from build123d import *

# Parameters (mm, degrees)
F1_W      = 200
F1_H      = 200
F1_W_2    = 191
F1_H_2    = 191
F2_DEPTH  = 94
F0_W      = 191
F0_H      = 191
F3_DEPTH  = 4
F6_W      = 20
F6_H      = 40
F9_DEPTH  = 35
F5_W      = 20
F5_H      = 40
F10_DEPTH = 35
F8_W      = 20
F8_H      = 40
F11_DEPTH = 35
F7_W      = 20
F7_H      = 40
F12_DEPTH = 35
F14_DEPTH = 25
F16_DEPTH = 25


with BuildPart() as f2:
    # F1 (on face) → F2 (new body)
    with BuildSketch(Plane.XY):
        Rectangle(F1_W, F1_H)
        Rectangle(F1_W_2, F1_H_2, mode=Mode.SUBTRACT)
    extrude(amount=F2_DEPTH)

    # F0 (on Top) → F3 (join)
    with BuildSketch(Plane.XY):
        Rectangle(F0_W, F0_H)
    extrude(amount=F3_DEPTH)

    # F6 (on offset) → F9 (join)
    with BuildSketch(Plane.XY.offset(39)):
        with Locations((-85.5, 75.5)):
            Rectangle(F6_W, F6_H)
    extrude(amount=-F9_DEPTH)

    # F5 (on offset) → F10 (join)
    with BuildSketch(Plane.XY.offset(39)):
        with Locations((-85.5, -75.5)):
            Rectangle(F5_W, F5_H)
    extrude(amount=-F10_DEPTH)

    # F8 (on offset) → F11 (join)
    with BuildSketch(Plane.XY.offset(39)):
        with Locations((85.5, -75.5)):
            Rectangle(F8_W, F8_H)
    extrude(amount=-F11_DEPTH)

    # F7 (on offset) → F12 (join)
    with BuildSketch(Plane.XY.offset(39)):
        with Locations((85.5, 75.5)):
            Rectangle(F7_W, F7_H)
    extrude(amount=-F12_DEPTH)

    # F13 (on face) → F14 (cut)
    with BuildSketch(Plane(origin=(-100, 0, 0), x_dir=(0, -1, 0), z_dir=(-1, 0, 0))):
        with BuildLine():
            Line((-67, 72), (-73, 72))
            ThreePointArc((-73, 72), (-77.949747, 69.949747), (-80, 65))
            Line((-80, 65), (-80, 52))
            Line((-80, 52), (-60, 52))
            Line((-60, 52), (-60, 65))
            ThreePointArc((-60, 65), (-62.050253, 69.949747), (-67, 72))
        make_face()
    extrude(amount=-F14_DEPTH, mode=Mode.SUBTRACT)

    # F15 (on face) → F16 (cut)
    with BuildSketch(Plane.YZ.offset(100)):
        with BuildLine():
            Line((-14, 62), (-16, 62))
            ThreePointArc((-16, 62), (-18.828427, 60.828427), (-20, 58))
            Line((-20, 58), (-20, 52))
            Line((-20, 52), (-10, 52))
            Line((-10, 52), (-10, 58))
            ThreePointArc((-10, 58), (-11.171573, 60.828427), (-14, 62))
        make_face()
    extrude(amount=-F16_DEPTH, mode=Mode.SUBTRACT)


solid = f2.part
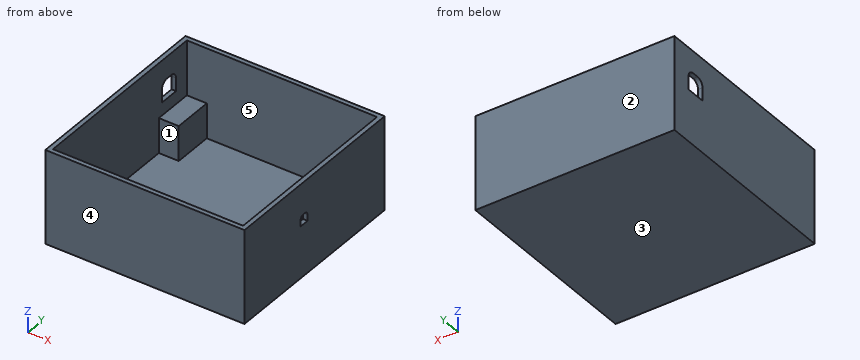
Input: part model. Units: mm. Frame: model coordinates. Face numbers are marked on the shaded views. A direction names the side the tool comes from. Give positions to 0.01 mm unless a question says otherwise; leave off trailing zeros. Write each loop counter-clockwise with the first axis right and the second up, starting at its lowest first coordinate (ties: lowest second). Pieces come first, ordered by that corner, then holes. Notation, with made-up numbers: M -26.5,-38.75 L 27.5,-38.75 A31 ccw 27.5,-13.75 Z; hole C 34,48 d2. An arc over 180 degrees is marked long. Use one line per item in the form item = value.
1. First-contact query: P1, Ø6, axis at x = -27, y = 78, coming from the +Z side; P2, Ø6, axis at x = -85.5, y = 83, coming from the +Z side. Flat tips, straight axial feed; report the tip coordinate or a pass-through.
Outcome:
P1 = 4
P2 = 39
2. Ray query, L1, parallel to X at y = 76.5, z = 38; L2, parallel to Y at x = 60.5, z = 36.5. Return the intervals inside material, ascending.
Outcome:
L1 = -100 to -75.5, 75.5 to 100
L2 = -100 to -95.5, 95.5 to 100
3. Cut plane A-A on z = 19. Return loops of the section in (x, y).
Outcome:
outline = M -100,-100 L 100,-100 L 100,100 L -100,100 Z; hole M -95.5,-55.5 L -75.5,-55.5 L -75.5,-95.5 L 75.5,-95.5 L 75.5,-55.5 L 95.5,-55.5 L 95.5,55.5 L 75.5,55.5 L 75.5,95.5 L -75.5,95.5 L -75.5,55.5 L -95.5,55.5 Z
4. Mould query, pull axis Y, two halves, no side actions, for the marked faces 1, 2 and 3. Classes: released by +Y, released by -Y, zero draft, split by the parting line, or undercut.
Outcome:
face_1 = undercut
face_2 = released by +Y
face_3 = zero draft
5. Cut plane C-C on y = -63. Return loops of the section in (x, z).
Outcome:
outline = M -100,0 L 100,0 L 100,94 L 95.5,94 L 95.5,39 L 75.5,39 L 75.5,4 L -75.5,4 L -75.5,39 L -95.5,39 L -95.5,94 L -100,94 Z
6. Cut plane B-B on x = 83.5. Return loops of the section in (y, z), and give its area (3 significant figures).
Outcome:
outline = M -100,0 L 100,0 L 100,94 L 95.5,94 L 95.5,39 L 55.5,39 L 55.5,4 L -55.5,4 L -55.5,39 L -95.5,39 L -95.5,94 L -100,94 Z
area = 4,410 mm²
7. Cut plane D-D on z = 83.5. Return loops of the section in (x, y).
Outcome:
outline = M -100,-100 L 100,-100 L 100,100 L -100,100 Z; hole M -95.5,-95.5 L 95.5,-95.5 L 95.5,95.5 L -95.5,95.5 Z
8. Reachability of the marked faces 4 and 5 from +Z, -Z, +X, -X, +Y, -Y: full face, straight path, thin tool, end or side. Return the list, or none.
Outcome:
face_4 = +Z, -Z, +X, -X, -Y
face_5 = +Z
